Autodesk Inventor part; units mm, degrees
ref_plane "YZ Plane" through (0, 0, 0) normal (1, 0, 0) x (0, 1, 0)
ref_plane "XZ Plane" through (0, 0, 0) normal (0, 1, 0) x (-1, 0, 0)
ref_plane "XY Plane" through (0, 0, 0) normal (0, 0, 1) x (1, 0, 0)
sketch "Sketch1" plane through (0, 0, 0) normal (1, 0, 0) x (0, 1, 0)
  line L0 (0, 0) -> (32.8422, 0)
  line L1 (32.8422, 0) -> (32.8422, 31.75)
  line L2 (32.8422, 31.75) -> (0, 31.75)
  line L3 (0, 31.75) -> (0, 0)
  dimension "d0" = 32.8422
  dimension "d1" = 31.75
extrude "Extrusion1" add sketch "Sketch1" along normal blind 127
sketch "Sketch2" plane through (0, 32.8422, 31.75) normal (0, 1, 0) x (1, 0, 0)
  line L0 (0, 0) -> (127, 0)
  line L1 (0, 31.75) -> (0, 0)
  point P0 (19.05, 6.35)
  point P1 (99.05, 6.35)
  dimension "d4" = 0
  dimension "d5" = 6.35
  dimension "d6" = 80
  dimension "d7" = 19.05
hole "Hole1" at (19.05, 32.8422, 25.4) at (99.05, 32.8422, 25.4) direction (0, -1, 0) diameter 3.175 end through all
sketch "Sketch3" plane through (127, 0, 0) normal (1, 0, 0) x (0, 0, -1)
  line L0 (-31.75, 32.8422) -> (0, 32.8422)
  line L1 (0, 32.8422) -> (0, 0)
  line L2 (0, 0) -> (-31.75, 0)
  line L3 (-31.75, 0) -> (-31.75, 32.8422)
  line L4 (0, 32.8422) -> (-31.75, 32.8422)
  line L5 (-31.75, 32.8422) -> (-31.75, 0)
  dimension "d15" = 0
  dimension "d16" = 0
extrude "Extrusion2" add sketch "Sketch3" along normal blind 25.4
sketch "Sketch4" plane through (0, 0, 0) normal (-1, 0, 0) x (0, 0, 1)
  line L0 (0, 32.8422) -> (31.75, 32.8422)
  line L1 (0, 32.8422) -> (31.75, 32.8422)
  line L2 (31.75, 32.8422) -> (31.75, 1.0922)
  line L3 (31.75, 1.0922) -> (0, 1.0922)
  line L4 (0, 1.0922) -> (0, 32.8422)
  point P0 (0, 0)
extrude "Extrusion3" add sketch "Sketch4" along normal blind 25.4
properties part number "StandoffBlocks"
Check sheet for the modelled part. Datum: model origin and axes. Units: mm. A direction names the side the tool comes from. Round coordinates to 2 decimals unless told otherwise and drop trailing zeros. Write each loop counter-clockwise with the first axis right and the second up, starting at its lowest first coordinate (ties: lowest second). Pieces come first, ordered by that corner, then holes. Notation, with made-up numbers: (-13.5, 6) - (39.5, 6) arc R27 ccw to (39.5, 39) - close; hole circle Ø3 at (-13.5, -17). An arc over 180 degrees is marked (long way). Return JSON: item names as keys, results as strings.
Q1. Cross-section at B-B (z = 25.4). Record the boundary of the cut face in (x, y), then the cut area to 3 significant figures.
Returned:
{"outline": "(-25.4, 1.09) - (0, 1.09) - (0, 0) - (17.46, 0) - (17.46, 32.84) - (-25.4, 32.84) - close; (20.64, 0) - (97.46, 0) - (97.46, 32.84) - (20.64, 32.84) - close; (100.64, 0) - (152.4, 0) - (152.4, 32.84) - (100.64, 32.84) - close", "area": "5,600 mm²"}
Q2. Draft check along Z on faces 3 (the flat face through (65, 16, 0)), 4 (the flat face through (65, 17, 31.75)), 5 (the cylindrical face through (98.573, 16.191, 26.914)), 6 (the flat face through (152.4, 17, 16)). Enter one of: released by +Z, released by -Z, zero draft, split by the parting line, or undercut.
Returned:
{"face 3": "released by -Z", "face 4": "released by +Z", "face 5": "undercut", "face 6": "zero draft"}
Q3. Access from +Z, -Z, +X, -X, +Y, -Y to the whole of each face (thin tool, end or side, straight path). Record for faces 1 (the flat face through (-13, 1.092, 16)), 2 (the cylindrical face through (18.573, 16.191, 26.914)).
Returned:
{"face 1": "+Z, -Z, -X, -Y", "face 2": "+Y, -Y"}
Q4. Depth check by flat-ended pin: P1, Ø5, axis at x = 116, z = 11.5, coming from the -Y side; P2, Ø2.5, axis at x = 19.05, z = 25.4, coming from the -Y side; P3, Ø0.5, axis at y = 0.5, z = 19, coming from the -X side; P4, Ø2, axis at x = -4, z = 16, coming from the -Y side. Enter the tip coordinate at first touch or a pass-through.
Returned:
{"P1": "stops at y = 0", "P2": "passes through", "P3": "stops at x = 0", "P4": "stops at y = 1.09"}
Q5. Cross-section at A-A (x = 19.05). Record the boundary of the cut face in (y, z).
Returned:
{"outline": "(0, 0) - (32.84, 0) - (32.84, 23.81) - (0, 23.81) - close; (0, 26.99) - (32.84, 26.99) - (32.84, 31.75) - (0, 31.75) - close"}
Q6. Scan lines: L1, parallel to X at y = 24, z = 25.4; L2, parallel to Z at x = 99, y = 11; L3, parallel to Y at x = -17, z = 25.5. Record each from-to range of solid material in increasing order. Write a range as from..to.
Returned:
{"L1": "x = -25.4..17.46, 20.64..97.46, 100.64..152.4", "L2": "z = 0..23.81, 26.99..31.75", "L3": "y = 1.09..32.84"}
